Design review of the part built by this model. Coordinates are the model's own, in mm. A direction names the side the tool comes from. Round coordinates to 2 decimals unless told otherwise and drop trailing zeros. Loops run counter-clockwise (first coordinate to the right, second up) from the corner with the lowest first, then second, coordinate; pieces in that order, holes last. Notation, with made-up numbers: M 20,-25 L 76,-25 A34 cw 76,8 Z; hole C -21,45 d5. An arc over 180 degrees is marked long. One line per item, written item: value. Start each with the question number.
Item 1: We need section D-D (y = 122). Write out the cut boundary in (x, z).
Item 2: We need section A-A (y = 93.5). Write out the cut boundary in (x, z).
Item 3: Mouldability with a two-part tool opening along X and no side actions: class faces 3 (the flat face through (95, 50, 3)), 4 (the cylindrical face through (274.297, 153.986, 2.958)), 5 (the cylindrical face through (5.703, 6.014, 2.958)) as released by +X, released by -X, zero draft, split by the parting line, or undercut.
Item 4: For faces 1 (the cylindrical face through (6.014, 154.297, 2.958)), 2 (the flat face through (152, 44.014, 3)), list the 3-axis set-ups (+Z, -Z, +X, -X, +Y, -Y) from which the entire face can be reached by the end or side of a thin tool; tool diameter is ignored.
Item 5: We need section C-C (z = 4). Write out the cut boundary in (x, y).
Item 6: Clearance check with a flat-ended pin moving along its axis: pin 1 (1.8 mm diameter, centred on y = 18, z = 4.5, fed in from -X). State where the tip first meets the part, or that it passes through.
Item 7: For line 1 along Y through (x, z) = (94, 5.3); line 2 along Y through (x, z) = (181.5, 3.35); line 3 along Y through (x, z) = (49, 2.6), list the stretches that pass through material, from the lowest coordinate up.
Item 8: We need section B-B (x = 134). Write out the cut boundary in (y, z).
from build123d import *

# Parameters (mm, degrees)
BOSS_EXTRUDE1_DEPTH = 6
SKETCH2_W           = 215
SKETCH2_H           = 20
CUT_EXTRUDE1_DEPTH  = 6


with BuildPart() as part:
    # Sketch1 → Boss-Extrude1 (new body)
    with BuildSketch(Plane.XY):
        with BuildLine():
            Line((20, 0), (260, 0))
            ThreePointArc((260, 0), (274.142135624, 5.857864376), (280, 20))
            Line((280, 20), (280, 140))
            ThreePointArc((280, 140), (274.142135624, 154.142135624), (260, 160))
            Line((260, 160), (20, 160))
            ThreePointArc((20, 160), (5.857864376, 154.142135624), (0, 140))
            Line((0, 140), (0, 20))
            ThreePointArc((0, 20), (5.857864376, 5.857864376), (20, 0))
        make_face()
    extrude(amount=BOSS_EXTRUDE1_DEPTH)

    # Sketch2 → Cut-Extrude1 (cut)
    with BuildSketch(Plane.XY.offset(6)):
        with Locations((140, 125)):
            Rectangle(SKETCH2_W, SKETCH2_H)
        Polygon((70, 89.013901834), (185, 89.013901834), (185, 101.513901834), (210, 101.513901834), (210, 56.513901834), (185, 56.513901834), (185, 69.013901834), (70, 69.013901834), align=None)
        Polygon((95, 56.513901834), (95, 44.013901834), (210, 44.013901834), (210, 24.013901834), (95, 24.013901834), (95, 11.513901834), (70, 11.513901834), (70, 56.513901834), align=None)
    extrude(amount=-CUT_EXTRUDE1_DEPTH, mode=Mode.SUBTRACT)


solid = part.part
A:
1. outline: M 0,0 L 32.5,0 L 32.5,6 L 0,6 Z; M 247.5,0 L 280,0 L 280,6 L 247.5,6 Z
2. outline: M 0,0 L 185,0 L 185,6 L 0,6 Z; M 210,0 L 280,0 L 280,6 L 210,6 Z
3. face 3: undercut
3. face 4: released by +X
3. face 5: released by -X
4. face 1: +Z, -Z, -X, +Y
4. face 2: +Z, -Z
5. outline: M 0,20 A20 ccw 20,0 L 260,0 A20 ccw 280,20 L 280,140 A20 ccw 260,160 L 20,160 A20 ccw 0,140 Z; hole M 32.5,115 L 247.5,115 L 247.5,135 L 32.5,135 Z; hole M 70,11.51 L 95,11.51 L 95,24.01 L 210,24.01 L 210,44.01 L 95,44.01 L 95,56.51 L 70,56.51 Z; hole M 70,69.01 L 185,69.01 L 185,56.51 L 210,56.51 L 210,101.51 L 185,101.51 L 185,89.01 L 70,89.01 Z
6. pin 1: x = 0.03
7. line 1: 0 to 11.51, 56.51 to 69.01, 89.01 to 115, 135 to 160
7. line 2: 0 to 24.01, 44.01 to 69.01, 89.01 to 115, 135 to 160
7. line 3: 0 to 115, 135 to 160
8. outline: M 0,0 L 24.01,0 L 24.01,6 L 0,6 Z; M 44.01,0 L 69.01,0 L 69.01,6 L 44.01,6 Z; M 89.01,0 L 115,0 L 115,6 L 89.01,6 Z; M 135,0 L 160,0 L 160,6 L 135,6 Z
